Autodesk Inventor part; units mm, degrees
ref_plane "YZ Plane" through (0, 0, 0) normal (1, 0, 0) x (0, 1, 0)
ref_plane "XZ Plane" through (0, 0, 0) normal (0, 1, 0) x (-1, 0, 0)
ref_plane "XY Plane" through (0, 0, 0) normal (0, 0, 1) x (1, 0, 0)
sketch "skirt" plane through (0, 0, 0) normal (0, 0, 1) x (1, 0, 0)
  circle A0 centre (5.0031, 25.9038) radius 4.7625
  line L0 (24.0531, -167.7712) -> (24.0531, 181.4788)
  line L1 (-25.1594, 145.2504) -> (-25.1594, -131.5428)
  circle A1 centre (11.3531, 133.8538) radius 2.1844
  arc A2 (24.0531, 181.4788) -> (20.8781, 184.6538) centre (20.8781, 181.4788) ccw
  line L2 (20.8781, 184.6538) -> (-4.6437, 184.6538)
  line L3 (-24.646, 147.7518) -> (-10.4803, 180.8052)
  arc A3 (-4.6437, 184.6538) -> (-10.4803, 180.8052) centre (-4.6437, 178.3038) ccw
  arc A4 (-24.646, 147.7518) -> (-25.1594, 145.2504) centre (-18.8094, 145.2504) ccw
  line L4 (-24.646, -134.0442) -> (-10.4803, -167.0976)
  line L5 (-4.6437, -170.9462) -> (20.8781, -170.9462)
  arc A5 (20.8781, -170.9462) -> (24.0531, -167.7712) centre (20.8781, -167.7712) ccw
  arc A6 (-25.1594, -131.5428) -> (-24.646, -134.0442) centre (-18.8094, -131.5428) ccw
  circle A7 centre (11.3531, -120.1462) radius 2.1844
  arc A8 (-10.4803, -167.0976) -> (-4.6437, -170.9462) centre (-4.6437, -164.5962) ccw
  circle A9 centre (5.0031, 102.1038) radius 4.7625
  circle A10 centre (5.0031, 76.7038) radius 4.7625
  circle A11 centre (5.0031, 64.0038) radius 4.7625
  circle A12 centre (5.0031, 38.6038) radius 4.7625
  circle A13 centre (5.0031, 0.5038) radius 4.7625
  circle A14 centre (11.3531, -31.2462) radius 2.1844
  circle A15 centre (5.0031, -62.9962) radius 4.7625
  circle A16 centre (5.0031, -88.3962) radius 4.7625
  circle A17 centre (5.0031, 89.4038) radius 2.1844
  point P0 (-0.9322, -0.2017)
  point P1 (5.0031, 51.3038)
  point P2 (-25.1594, 146.5538)
  point P3 (-25.1594, -132.8462)
  point P4 (5.0031, -12.1962)
  point P5 (5.0031, 13.2038)
  dimension "d0" = 279.4
  dimension "d1" = 49.2125
  dimension "d2" = 3.175
  dimension "d3" = 113.199
  dimension "d4" = 113.199
  dimension "d5" = 6.35
  dimension "d7" = 9.525
  dimension "d13" = 50.8
  dimension "d14" = 50.8
  dimension "d15" = 9.525
  dimension "d16" = 4.3688
  dimension "d17" = 31.75
  dimension "d18" = 4.3688
sketch "Sketch1" plane through (0, 0, 0) normal (1, 0, 0) x (0, 1, 0)
  circle A0 centre (-6.35, -107.95) radius 4.7625
  line L0 (12.7, -301.625) -> (12.7, 47.625)
  line L1 (-36.5125, 11.3966) -> (-36.5125, -265.3966)
  circle A1 centre (0, 0) radius 2.1844
  arc A2 (12.7, 47.625) -> (9.525, 50.8) centre (9.525, 47.625) ccw
  line L2 (9.525, 50.8) -> (-15.9968, 50.8)
  line L3 (-35.9991, 13.898) -> (-21.8333, 46.9514)
  arc A3 (-15.9968, 50.8) -> (-21.8333, 46.9514) centre (-15.9968, 44.45) ccw
  arc A4 (-35.9991, 13.898) -> (-36.5125, 11.3966) centre (-30.1625, 11.3966) ccw
  line L4 (-35.9991, -267.898) -> (-21.8333, -300.9514)
  line L5 (-15.9968, -304.8) -> (9.525, -304.8)
  arc A5 (9.525, -304.8) -> (12.7, -301.625) centre (9.525, -301.625) ccw
  arc A6 (-36.5125, -265.3966) -> (-35.9991, -267.898) centre (-30.1625, -265.3966) ccw
  circle A7 centre (0, -254) radius 2.1844
  arc A8 (-21.8333, -300.9514) -> (-15.9968, -304.8) centre (-15.9968, -298.45) ccw
  circle A9 centre (-6.35, -31.75) radius 4.7625
  circle A10 centre (-6.35, -57.15) radius 4.7625
  circle A11 centre (-6.35, -69.85) radius 4.7625
  circle A12 centre (-6.35, -95.25) radius 4.7625
  circle A13 centre (-6.35, -133.35) radius 4.7625
  circle A14 centre (0, -165.1) radius 2.1844
  circle A15 centre (-6.35, -196.85) radius 4.7625
  circle A16 centre (-6.35, -222.25) radius 4.7625
  circle A17 centre (-6.35, -44.45) radius 2.1844
extrude "Extrusion1" add sketch "Sketch1" along normal blind 1.5875
properties part number "Skirt" material "Acetal Resin, White"
The model under review builds one solid part; all positions refer to its coordinate system, in mm. Give positions to 0.01 mm unless a question says otherwise; leave off trailing zeros. Write each loop counter-clockwise with the first axis right and the second up, starting at its lowest first coordinate (ties: lowest second). Pieces come first, ordered by that corner, then holes. Notation, with made-up numbers: M 21.25,39.5 L 74.25,39.5 A16 cw 74.25,55.5 Z; hole C 42.5,13.5 d3. An arc over 180 degrees is marked long. Answer in a Markdown table with one row per item.
Item 1: For line 1 along Z through (x, y) = (0.4, 0); line 2 along Y through (x, z) = (0.85, -165.1); line 3 along Y through (x, z) = (1, -194.5), list the stretches that pass through material, from the lowest coordinate up.
Check sheet entries:
| item | result |
|---|---|
| line 1 | -304.8 to -256.18, -251.82 to -167.28, -162.92 to -2.18, 2.18 to 50.8 |
| line 2 | -36.51 to -2.18, 2.18 to 12.7 |
| line 3 | -36.51 to -10.49, -2.21 to 12.7 |
Item 2: Add section A-A on x = 1.1. State how many separate pieces and enclosed holes the cut face has, plus the area to 3 significant figures.
Check sheet entries:
| item | result |
|---|---|
| separate pieces | 1 |
| enclosed holes | 12 |
| area | 16,200 mm2 |
Item 3: Add section B-B on z = -107.95. Give the boundary of the cut face in (x, y).
Check sheet entries:
| item | result |
|---|---|
| outline | M 0,-36.51 L 1.59,-36.51 L 1.59,-11.11 L 0,-11.11 Z; M 0,-1.59 L 1.59,-1.59 L 1.59,12.7 L 0,12.7 Z |
Item 4: Add section C-C on y = -31. Give the boundary of the cut face in (x, z), plus the area to 3 significant figures.
Check sheet entries:
| item | result |
|---|---|
| outline | M 0,-279.56 L 1.59,-279.56 L 1.59,25.56 L 0,25.56 Z |
| area | 484 mm2 |
Item 5: Draft analysis for pull direction Y (two halves, no side actions). For faces 1 (the face through (0.78, -6.97, -99.97)), 2 (the face through (1.588, -12, -125)), 3 (the face through (0.783, -29.015, -284.193)), state which applies: +Y half, -Y half, draft (parallel to the pull), parting line (faces both ways), or undercut.
Check sheet entries:
| item | result |
|---|---|
| face 1 | undercut |
| face 2 | draft |
| face 3 | -Y half |
